Build history of the part. All positions in model axes, mm. A direction names the side the tool comes from. Coordinates: 2 decimals unless noted, no trailing zeros. Loops run counter-clockwise (first coordinate to the right, second up) from the corner with the lowest first, then second, coordinate; pieces in that order, holes last. Notation, with made-up numbers: (62.5, 31) - (101.5, 31) arc R25 ccw to (101.5, 53) - close; hole circle Ø3 at (13, 35). An arc over 180 degrees is marked (long way). One line per item, written item: value.
```python
from build123d import *

# Parameters (mm, degrees)
SKETCH1_R           = 150
BOSS_EXTRUDE3_DEPTH = 25
SKETCH6_R           = 300
SKETCH6_R_2         = 150
BOSS_EXTRUDE6_DEPTH = 200
SKETCH9_R           = 60
BOSS_EXTRUDE8_DEPTH = 254.189683417
SKETCH10_W          = 145.864440971
SKETCH10_H          = 70
SKETCH10_W_2        = 154.135559029
CUT_EXTRUDE1_DEPTH  = 300


with BuildPart() as part:
    # Sketch1 → Boss-Extrude3 (new body, symmetric)
    with BuildSketch(Plane.XY):
        with BuildLine():
            Line((179.794520548, 127.397260274), (-70.205479452, 127.397260274))
            Line((-70.205479452, 127.397260274), (-70.205479452, -127.397260274))
            Line((-70.205479452, -127.397260274), (179.794520548, -127.397260274))
            Line((179.794520548, -127.397260274), (1084.183927904, -291.571850847))
            Line((1084.183927904, -291.571850847), (1118.418389374, -297.786462219))
            ThreePointArc((1118.418389374, -297.786462219), (1454.794520548, 0), (1118.418389374, 297.786462219))
            Line((1118.418389374, 297.786462219), (1084.183927904, 291.571850847))
            Line((1084.183927904, 291.571850847), (179.794520548, 127.397260274))
        make_face()
        with Locations((1154.794520548, 0)):
            Circle(SKETCH1_R, mode=Mode.SUBTRACT)
    boss_extrude3 = extrude(amount=BOSS_EXTRUDE3_DEPTH, both=True)

    # Sketch6 → Boss-Extrude6 (add)
    with BuildSketch(Plane.XY.offset(25)):
        with Locations(Location((1154.794520548, 0, 0), (0, 0, 256.386646044))):  # turned: the seam where the file's is
            Circle(SKETCH6_R)
        with Locations((1154.794520548, 0)):
            Circle(SKETCH6_R_2, mode=Mode.SUBTRACT)
    boss_extrude6 = extrude(amount=BOSS_EXTRUDE6_DEPTH)

    # Mirror1: Boss-Extrude3, Boss-Extrude6 across plane
    add(boss_extrude3.mirror(Plane.XY.offset(-25)))
    add(boss_extrude6.mirror(Plane.XY.offset(-25)))

    # Sketch9 → Boss-Extrude8 (add)
    with BuildSketch(Plane(origin=(0, 127.397260274, 0), x_dir=(1, 0, 0), z_dir=(0, 1, 0))):
        with BuildLine():
            Line((179.794520548, 75), (179.794520548, 220.864440971))
            ThreePointArc((179.794520548, 220.864440971), (54.794520548, 345.864440971), (-70.205479452, 220.864440971))
            Line((-70.205479452, 220.864440971), (-70.205479452, 75))
            Line((-70.205479452, 75), (179.794520548, 75))
        make_face()
        with Locations(Location((54.794520548, 220.864440971, 0), (0, 0, 270))):  # turned: the seam where the file's is
            Circle(SKETCH9_R, mode=Mode.SUBTRACT)
    extrude(amount=-BOSS_EXTRUDE8_DEPTH)

    # Sketch10 → Cut-Extrude1 (cut)
    with BuildSketch(Plane.ZY.offset(70.205479452)):
        with Locations((-147.932220486, -35)):
            Rectangle(SKETCH10_W, SKETCH10_H)
        with Locations((-297.932220486, -35)):
            Rectangle(SKETCH10_W_2, SKETCH10_H)
        with Locations((-297.932220486, 35)):
            Rectangle(SKETCH10_W_2, SKETCH10_H)
        with Locations((-147.932220486, 35)):
            Rectangle(SKETCH10_W, SKETCH10_H)
    extrude(amount=-CUT_EXTRUDE1_DEPTH, mode=Mode.SUBTRACT)


solid = part.part
```
Item 1: Drop flat-ended pins along their axis: P1, Ø12, axis at x = 605.5, y = -40.5, coming from the +Z side; P2, Ø1.5, axis at x = 681.5, z = -65.5, coming from the -Y side; P3, Ø17, axis at y = 112.5, z = -128.5, coming from the +X side. Give the stop position or say it passes through.
Check result:
P1: stops at z = 25
P2: stops at y = -218.61
P3: stops at x = 1436.19
Item 2: Cut at B-B, the plane z = -205. Write the cut outline in (x, y).
Check result:
outline: (-70.21, -126.79) - (-3.07, -126.79) - (-3.07, -70) - (-70.21, -70) - close; (-70.21, 70) - (-3.07, 70) - (-3.07, 127.4) - (-70.21, 127.4) - close; (112.66, -126.79) - (179.79, -126.79) - (179.79, -70) - (112.66, -70) - close; (112.66, 70) - (179.79, 70) - (179.79, 127.4) - (112.66, 127.4) - close; circle Ø600 at (1154.79, 0); hole circle Ø300 at (1154.79, 0)
Item 3: Cut at A-A, the plane y = 0. Write the cut outline in (x, z).
Check result:
outline: (-70.21, -75) - (854.79, -75) - (854.79, -275) - (1004.79, -275) - (1004.79, 225) - (854.79, 225) - (854.79, 25) - (-70.21, 25) - close; (1304.79, -275) - (1454.79, -275) - (1454.79, 225) - (1304.79, 225) - close
Item 4: Cut at D-D, the plane z = 157. Write the cut outline in (x, y), then the cut area to 3 significant figures.
Check result:
outline: circle Ø600 at (1154.79, 0); hole circle Ø300 at (1154.79, 0)
area: 212,000 mm^2
Item 5: Cut at C-C, the plane x = 1194. Write the cut outline in (y, z), then the cut area to 3 significant figures.
Check result:
outline: (-297.43, -275) - (-144.79, -275) - (-144.79, 225) - (-297.43, 225) - close; (144.79, -275) - (297.43, -275) - (297.43, 225) - (144.79, 225) - close
area: 153,000 mm^2
Item 6: Pull direction X, two halves, no side cores. Call faces 1 (the face through (-70.205, 2, -72)), 2 (the face through (18.29, 99.1, -268.48)), 3 (the face through (1126, 148, 225)): released by +X, released by -X, zero draft, split by the parting line, or undercut.
Check result:
face 1: released by -X
face 2: undercut
face 3: zero draft
Item 7: Tool access for faces 4 (the face through (179.795, -98, -147)), 5 (the face through (499, 4, -75)), 6 (the face through (53, 127.397, -122)): list every direction of +Z, -Z, +X, -X, +Y, -Y with a clear straight run to the whole face (end or side of a thin tool).
Check result:
face 4: -Z, +Y, -Y
face 5: -Z
face 6: +Z, -Z, -X, +Y
Item 8: Probe probe 1 along Z at (x, y) = (892.5, 96); probe 2 along Z at (x, y) = (582, -69.5); probe 3 along X at (y, z) = (-126, -225). List the from-to ranges inside material, lowest first. Write a range as from..to.
Check result:
probe 1: z = -275..225
probe 2: z = -75..25
probe 3: x = -70.14..-5.06, 114.65..179.73, 882.54..1073.41, 1236.18..1427.05
